```python
from build123d import *

# Parameters (mm, degrees)
F0_R     = 14.478
F1_DEPTH = 2.54
F0_R_2   = 17.5196905757
F2_DEPTH = 15.24


# Not quite as in the source:
# - a fillet or chamfer that OpenCascade refuses, or shapes differently, is made with other operations: its cross-section is extruded or revolved along the edge and cut away or added


with BuildPart() as f1:
    # F0 (on Front) → F1 (new body)
    with BuildSketch(Plane.XZ):
        Circle(F0_R)
    extrude(amount=F1_DEPTH)

    # F0 (on Front) → F2 (join)
    with BuildSketch(Plane.XZ):
        Circle(F0_R_2)
        Circle(F0_R, mode=Mode.SUBTRACT)
    extrude(amount=F2_DEPTH)

    # F3: fillet of radius 5.08 on 3 edges, made by hand

    # F3_s1 → F3_t2 (revolve, cut)
    with BuildSketch(Plane.XY):
        with BuildLine():
            ThreePointArc((12.4396905757, 0), (16.0317930242, -1.4878975516), (17.5196905757, -5.08))
            Line((17.5196905757, -5.08), (17.6212905757, -5.08))
            Line((17.6212905757, -5.08), (17.6212905757, 0.1016))
            Line((17.6212905757, 0.1016), (12.4396905757, 0.1016))
            Line((12.4396905757, 0.1016), (12.4396905757, 0))
        make_face()
    revolve(axis=Axis((0, 0, 0), (0, -1, 0)), mode=Mode.SUBTRACT)

    # F3_s3 → F3_t4 (revolve, cut)
    with BuildSketch(Plane.XY):
        with BuildLine():
            ThreePointArc((17.5196905757, -10.5868618448), (16.6918083937, -13.3664111001), (14.478, -15.24))
            Line((14.478, -15.24), (14.5187661885, -15.3330627631))
            ThreePointArc((14.5187661885, -15.3330627631), (15.9988452879, -15.3416), (17.5196905757, -15.3416))
            Line((17.5196905757, -15.3416), (17.6212905757, -15.24))
            Line((17.6212905757, -15.24), (17.6212905757, -10.5868618448))
            Line((17.6212905757, -10.5868618448), (17.5196905757, -10.5868618448))
        make_face()
    revolve(axis=Axis((0, -15.24, 0), (0, -1, 0)), mode=Mode.SUBTRACT)


solid = f1.part
```
Can you work these out from the model? Positions are in its coordinate system, mm. Coordinates: 2 decimals unless noted, no trailing zeros. Loops run counter-clockwise (first coordinate to the right, second up) from the corner with the lowest first, then second, coordinate; pieces in that order, holes last.
1) Imagine slicing it at B-B on x = 0. List the corners of the cut face in (y, z) for me.
2) Thinking about a two-plate mould opening in Z: for faces 1 (the cylindrical face through (16.7, -7.8, 5.3)), 2 (the cylindrical face through (-1.885, -8.801, 14.355)), 3 (the flat face through (0, 0, 0)), which applies, pulls with the +Z half, pulls with the -Z half, needs draft (parallel to the pull), parting line crosses it, or undercut?
3) Imagine slicing it at D-D on y = -12.5. List the corners of the cut face in (x, z) for me, plus the area to 3 significant figures.
4) Imagine slicing it at A-A on z = 0. List the corners of the cut face in (x, y) for me.
5) For pin 1 (1 mm diameter, centred on x = 14, z = 5, fed in from -Y); pin 2 (3 mm diameter, centred on x = -13, y = -13.5, fed in from -Z); pin 3 (1.5 mm diameter, centred on x = 14, z = 1.5, fed in from +Y); pin 4 (5 mm diameter, centred on y = -3.5, z = 7, fed in from +X), each with a flat end and sliding along its axis, tell me the tip position at first contact or that it passes through.
6) I need wall thicknesses on probe 1 along X at (y, z) = (-8.5, 0.5); probe 2 along Z at (x, y) = (0, -9); probe 3 along Y at (x, z) = (-2, -5.5). Which ranges of each line are inside material? Lowest first, please.
7) Imagine slicing it at C-C on y = -7.5. List the corners of the cut face in (x, z) for me.
Completed:
1. outline: (-15.24, -14.48) arc R5.08 ccw to (-10.59, -17.52) - (-5.08, -17.52) arc R5.08 ccw to (0, -12.44) - (0, 12.44) arc R5.08 ccw to (-5.08, 17.52) - (-10.59, 17.52) arc R5.08 ccw to (-15.24, 14.48) - (-2.54, 14.48) - (-2.54, -14.48) - close
2. face 1: parting line crosses it
2. face 2: undercut
2. face 3: needs draft
3. outline: circle Ø34.29 at (0, 0); hole circle Ø28.96 at (0, 0)
3. area: 265 mm2
4. outline: (-17.52, -10.59) arc R5.08 ccw to (-14.48, -15.24) - (-14.48, -2.54) - (14.48, -2.54) - (14.48, -15.24) arc R5.08 ccw to (17.52, -10.59) - (17.52, -5.08) arc R5.08 ccw to (12.44, 0) - (-12.44, 0) arc R5.08 ccw to (-17.52, -5.08) - close
5. pin 1: stops at y = -15.24
5. pin 2: stops at z = -12.39
5. pin 3: stops at y = -0.08
5. pin 4: stops at x = 16.84
6. probe 1: x = -17.51 to -14.47, 14.47 to 17.51
6. probe 2: z = -17.52 to -14.48, 14.48 to 17.52
6. probe 3: y = -2.54 to 0
7. outline: circle Ø35.04 at (0, 0); hole circle Ø28.96 at (0, 0)
